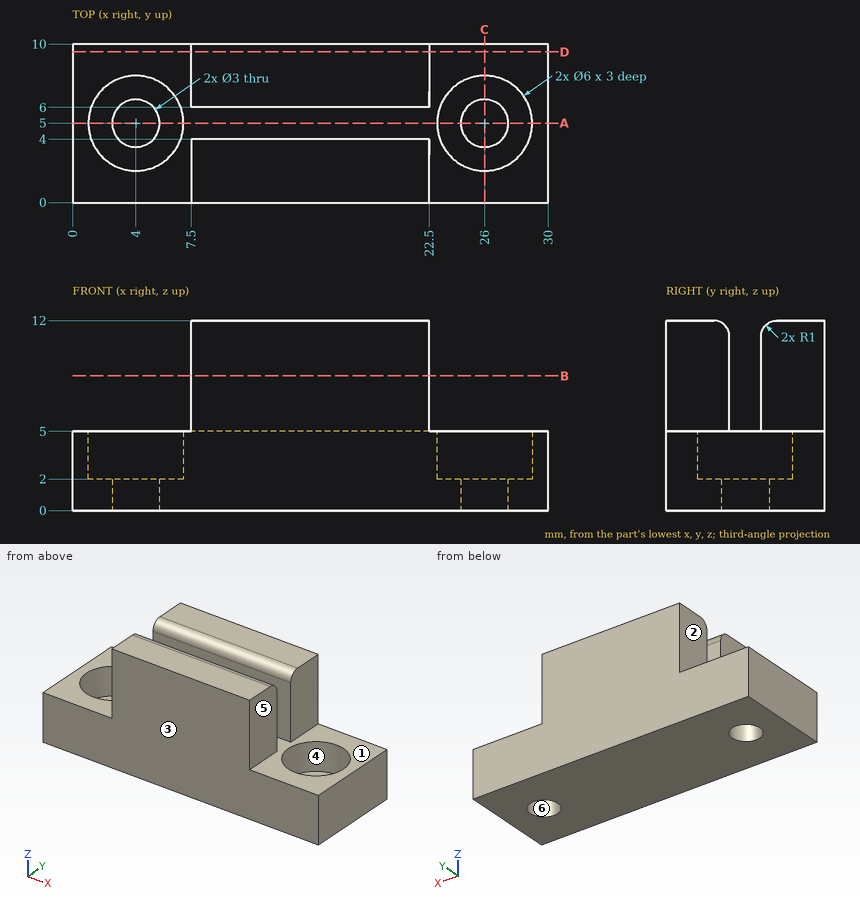
Here's the drawing with two shaded views (mm, measured from the low corner). I have some questions. A direction names the side the tool comes from. Give positions to 0.01 mm unless a question says otherwise; leave off trailing zeros. Loops run counter-clockwise (first coordinate to the right, second up) from the corner with the lowest first, then second, coordinate; pieces in that order, holes last. Notation, with made-up numbers: (48.5, -20) - (52.5, -20) arc R31 cw to (52.5, 10) - close; hole circle Ø6 at (-21, -5). An arc over 180 degrees is marked (long way). Return JSON: item names as keys, results as strings.
1. We'd pull the mould along Y, two halves only. Please class the marked faces 1, 2 and 3: +Y half, -Y half, draft (parallel to the pull), parting line (faces both ways), or undercut.
Output values:
{"face 1": "undercut", "face 2": "draft", "face 3": "-Y half"}
2. I want a section at A-A on y = 5. Please give me the cut outline in (x, z), and give its area (3 significant figures).
Output values:
{"outline": "(0, 0) - (2.5, 0) - (2.5, 2) - (1, 2) - (1, 5) - (0, 5) - close; (5.5, 0) - (24.5, 0) - (24.5, 2) - (23, 2) - (23, 5) - (7, 5) - (7, 2) - (5.5, 2) - close; (27.5, 0) - (30, 0) - (30, 5) - (29, 5) - (29, 2) - (27.5, 2) - close", "area": "102 mm²"}
3. I want a section at B-B on z = 8.5. Please give me the cut outline in (x, y), and give its area (3 significant figures).
Output values:
{"outline": "(7.5, 0) - (22.5, 0) - (22.5, 4) - (7.5, 4) - close; (7.5, 6) - (22.5, 6) - (22.5, 10) - (7.5, 10) - close", "area": "120 mm²"}
4. If I drill on line 1 (Y direction, x = 4, z = 1.3); line 2 (Y direction, x = 26, z = 3.55); line 3 (X direction, y = 6, z = 2.5), over which ranges is the centre line in solid material (lowest first)?
Output values:
{"line 1": "y = 0 to 3.5, 6.5 to 10", "line 2": "y = 0 to 2, 8 to 10", "line 3": "x = 0 to 1.17, 6.83 to 23.17, 28.83 to 30"}
5. I want a section at C-C on x = 26. Please give me the cut outline in (y, z), and give its area (3 significant figures).
Output values:
{"outline": "(0, 0) - (3.5, 0) - (3.5, 2) - (2, 2) - (2, 5) - (0, 5) - close; (6.5, 0) - (10, 0) - (10, 5) - (8, 5) - (8, 2) - (6.5, 2) - close", "area": "26.0 mm²"}
6. For the marked faces 4, 5 and 6, which set-ups out of +Z, -Z, +X, -X, +Y, -Y let a thin tool reach every point of the face, with its end or its side?
Output values:
{"face 4": "+Z", "face 5": "+Z, +X, +Y, -Y", "face 6": "+Z, -Z"}
7. I'm going to push flat-ended pins straight in: pin 1 Ø3 at (y, z) = (1.5, 10) entering from -X; pin 2 Ø5 at (y, z) = (1.5, 9.5) entering from +X; pin 3 Ø3.5 at (x, y) = (4, 5) entering from +Z. Where does each tip first touch, or does it pass through?
Output values:
{"pin 1": "stops at x = 7.5", "pin 2": "stops at x = 22.5", "pin 3": "stops at z = 2"}
8. I want a section at D-D on y = 9.5. Please give me the cut outline in (x, z), and give its area (3 significant figures).
Output values:
{"outline": "(0, 0) - (30, 0) - (30, 5) - (22.5, 5) - (22.5, 12) - (7.5, 12) - (7.5, 5) - (0, 5) - close", "area": "255 mm²"}
